Geometry: final body of the model. Coordinates: model frame, mm. Face numbers are marked on the shaded views. A direction names the side the tool comes from. Give positions to 0.01 mm unless a question says otherwise; leave off trailing zeros. Loops run counter-clockwise (first coordinate to the right, second up) from the corner with the lowest first, then second, coordinate; pieces in that order, holes last. Notation, with made-up numbers: (-38, 9) -> (11, 9) arc R31 ccw to (11, 36) -> close; hole circle Ø5 at (42.5, 86). An arc over 180 degrees is marked (long way). One line per item, written item: value. Start each with the question number.
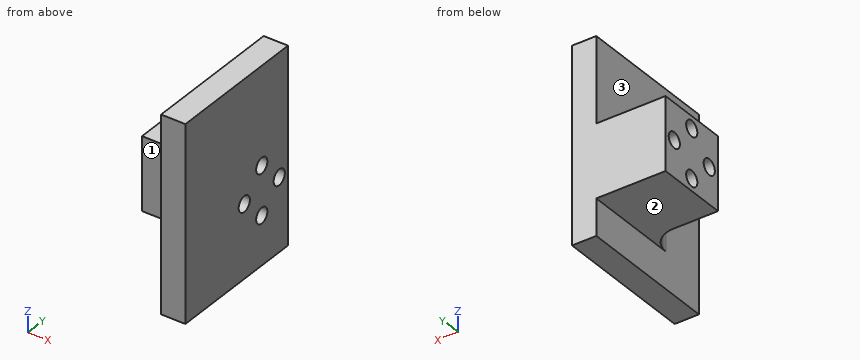
from build123d import *

# Parameters (mm, degrees)
BOSS_EXTRUDE1_DEPTH     = 5
CUT_EXTRUDE1_DEPTH      = 114.468057179
CUT_EXTRUDE1_DEPTH_BACK = 114.468057179
SKETCH3_R               = 1.6
SKETCH4_R               = 2.55
CUT_EXTRUDE2_DEPTH      = 10
SKETCH5_R               = 1.55
CUT_EXTRUDE3_DEPTH      = 114.468057179
SKETCH6_R               = 1.55
CUT_EXTRUDE4_DEPTH      = 114.468057179
SKETCH7_W               = 23
SKETCH7_H               = 110
BOSS_EXTRUDE2_DEPTH     = 5
SKETCH9_W               = 5
SKETCH9_H               = 40
BOSS_EXTRUDE4_DEPTH     = 33
SKETCH11_W              = 12
SKETCH11_H              = 12
CUT_EXTRUDE5_DEPTH      = 50
SKETCH12_R              = 1.6
CUT_EXTRUDE6_DEPTH      = 50
BOSS_EXTRUDE5_START     = 14.25
SKETCH13_W              = 15
SKETCH13_H              = 15
SKETCH13_R              = 1.6
BOSS_EXTRUDE5_DEPTH     = 14.25
SKETCH15_W              = 89.5
SKETCH15_H              = 3.65
CUT_EXTRUDE9_DEPTH      = 153.144667997
SKETCH18_W              = 13
SKETCH18_H              = 110
CUT_EXTRUDE10_DEPTH     = 134.005347637
FILLET5_R               = 5
SKETCH19_R              = 1.55
CUT_EXTRUDE11_DEPTH     = 5
CUT_EXTRUDE12_DEPTH     = 189.758900452


with BuildPart() as part:
    # Sketch1 → Boss-Extrude1 (new body)
    with BuildSketch(Plane(origin=(0, 0, 0), x_dir=(1, 0, 0), z_dir=(0, 1, 0))):
        Polygon((75, 85), (-75, 85), (-75, -25), (-45, -45), (-45, -80), (45, -80), (45, -45), (75, -25), align=None)
        Polygon((-18.5, -10), (-18.5, 10), (-7.5, 10), (-7.5, 50), (7.5, 50), (7.5, 10), (18.5, 10), (18.5, -10), align=None, mode=Mode.SUBTRACT)
    extrude(amount=BOSS_EXTRUDE1_DEPTH)

    # Sketch3 → Cut-Extrude1 (cut, two sides: drawn at the far end of the back side and taken through both)
    with BuildSketch(Plane(origin=(0, 5, 0), x_dir=(1, 0, 0), z_dir=(0, 1, 0)).offset(-CUT_EXTRUDE1_DEPTH_BACK)):
        with Locations(Location((-35, 20, 0), (0, 0, 270))):
            Circle(SKETCH3_R)
        with Locations(Location((-35, -20, 0), (0, 0, 270))):
            Circle(SKETCH3_R)
        with Locations(Location((35, -20, 0), (0, 0, 270))):
            Circle(SKETCH3_R)
        with Locations(Location((35, 20, 0), (0, 0, 270))):
            Circle(SKETCH3_R)
    extrude(amount=CUT_EXTRUDE1_DEPTH + CUT_EXTRUDE1_DEPTH_BACK, mode=Mode.SUBTRACT)

    # Sketch4 → Cut-Extrude2 (cut)
    with BuildSketch(Plane(origin=(0, 5, 0), x_dir=(1, 0, 0), z_dir=(0, 1, 0))):
        with Locations(Location((-65, 66, 0), (0, 0, 270))):
            Circle(SKETCH4_R)
        with Locations(Location((65, -4, 0), (0, 0, 270))):
            Circle(SKETCH4_R)
        with Locations(Location((-65, -4, 0), (0, 0, 270))):
            Circle(SKETCH4_R)
        with Locations(Location((65, 66, 0), (0, 0, 270))):
            Circle(SKETCH4_R)
    extrude(amount=-CUT_EXTRUDE2_DEPTH, mode=Mode.SUBTRACT)

    # Sketch5 → Cut-Extrude3 (cut, through all)
    with BuildSketch(Plane(origin=(0, 5, 0), x_dir=(1, 0, 0), z_dir=(0, 1, 0))):
        with Locations(Location((-39, -75, 0), (0, 0, 270))):
            Circle(SKETCH5_R)
        with Locations(Location((39, -75, 0), (0, 0, 90))):
            Circle(SKETCH5_R)
        with Locations(Location((-39, -50, 0), (0, 0, 270))):
            Circle(SKETCH5_R)
        with Locations(Location((39, -50, 0), (0, 0, 90))):
            Circle(SKETCH5_R)
    extrude(amount=-CUT_EXTRUDE3_DEPTH, mode=Mode.SUBTRACT)

    # Sketch6 → Cut-Extrude4 (cut, through all)
    with BuildSketch(Plane(origin=(0, 5, 0), x_dir=(1, 0, 0), z_dir=(0, 1, 0))):
        with Locations(Location((62.5, 80, 0), (0, 0, 270))):
            Circle(SKETCH6_R)
        with Locations(Location((-62.5, 80, 0), (0, 0, 90))):
            Circle(SKETCH6_R)
    extrude(amount=-CUT_EXTRUDE4_DEPTH, mode=Mode.SUBTRACT)

    # Sketch7 → Boss-Extrude2 (add)
    with BuildSketch(Plane(origin=(0, 5, 0), x_dir=(1, 0, 0), z_dir=(0, 1, 0))):
        with Locations((-86.5, 30)):
            Rectangle(SKETCH7_W, SKETCH7_H)
        with Locations((86.5, 30)):
            Rectangle(SKETCH7_W, SKETCH7_H)
    extrude(amount=-BOSS_EXTRUDE2_DEPTH)

    # Sketch9 → Boss-Extrude4 (add)
    with BuildSketch(Plane(origin=(0, 5, 0), x_dir=(1, 0, 0), z_dir=(0, 1, 0))):
        with Locations((-42.25, -5)):
            Rectangle(SKETCH9_W, SKETCH9_H)
        with Locations((42.25, -5)):
            Rectangle(SKETCH9_W, SKETCH9_H)
    extrude(amount=BOSS_EXTRUDE4_DEPTH)

    # Sketch11 → Cut-Extrude5 (cut)
    with BuildSketch(Plane(origin=(0, 5, 0), x_dir=(1, 0, 0), z_dir=(0, 1, 0))):
        with Locations((-67, 18.305755671)):
            Rectangle(SKETCH11_W, SKETCH11_H)
        with Locations((67, 18.305755671)):
            Rectangle(SKETCH11_W, SKETCH11_H)
    extrude(amount=-CUT_EXTRUDE5_DEPTH, mode=Mode.SUBTRACT)

    # Sketch12 → Cut-Extrude6 (cut)
    with BuildSketch(Plane.ZY.offset(44.75)):
        with Locations((0, 31.85)):
            Circle(SKETCH12_R)
        with Locations((5, 26.85)):
            Circle(SKETCH12_R)
        with Locations((0, 21.85)):
            Circle(SKETCH12_R)
        with Locations((-5, 26.85)):
            Circle(SKETCH12_R)
    cut_extrude6 = extrude(amount=-CUT_EXTRUDE6_DEPTH, mode=Mode.SUBTRACT)

    # Sketch13 → Boss-Extrude5 (add)
    with BuildSketch(Plane.ZY.offset(44.75).offset(BOSS_EXTRUDE5_START)):
        with Locations((0, 26.85)):
            Rectangle(SKETCH13_W, SKETCH13_H)
        with Locations((0, 31.85)):
            Circle(SKETCH13_R, mode=Mode.SUBTRACT)
        with Locations((5, 26.85)):
            Circle(SKETCH13_R, mode=Mode.SUBTRACT)
        with Locations((-5, 26.85)):
            Circle(SKETCH13_R, mode=Mode.SUBTRACT)
        with Locations((0, 21.85)):
            Circle(SKETCH13_R, mode=Mode.SUBTRACT)
    boss_extrude5 = extrude(amount=-BOSS_EXTRUDE5_DEPTH)

    # Mirror2: Cut-Extrude6 across plane
    add(cut_extrude6.mirror(Plane.ZY), mode=Mode.SUBTRACT)

    # Mirror3: Boss-Extrude5 across plane
    add(boss_extrude5.mirror(Plane.ZY))

    # Sketch15 → Cut-Extrude9 (cut, through all)
    with BuildSketch(Plane.XY.offset(25)):
        with Locations((0, 36.175)):
            Rectangle(SKETCH15_W, SKETCH15_H)
    extrude(amount=-CUT_EXTRUDE9_DEPTH, mode=Mode.SUBTRACT)

    # Sketch18 → Cut-Extrude10 (cut, through all)
    with BuildSketch(Plane(origin=(0, 5, 0), x_dir=(1, 0, 0), z_dir=(0, 1, 0))):
        with Locations((-91.5, 30)):
            Rectangle(SKETCH18_W, SKETCH18_H)
        with Locations((91.5, 30)):
            Rectangle(SKETCH18_W, SKETCH18_H)
    extrude(amount=-CUT_EXTRUDE10_DEPTH, mode=Mode.SUBTRACT)

    # Fillet5
    fillet5_edges = [part.edges().sort_by_distance(p)[0] for p in [
        (-44.75, 19.35, 0),
        (44.75, 19.35, 0),
    ]]
    fillet(fillet5_edges, radius=FILLET5_R)

    # Sketch19 → Cut-Extrude11 (cut)
    with BuildSketch(Plane(origin=(0, 5, 0), x_dir=(1, 0, 0), z_dir=(0, 1, 0))):
        with Locations(Location((55, 34.5, 0), (0, 0, 270))):
            Circle(SKETCH19_R)
        with Locations(Location((25, 34.5, 0), (0, 0, 270))):
            Circle(SKETCH19_R)
        with Locations(Location((25, 44.5, 0), (0, 0, 270))):
            Circle(SKETCH19_R)
        with Locations(Location((55, 44.5, 0), (0, 0, 270))):
            Circle(SKETCH19_R)
    cut_extrude11 = extrude(amount=-CUT_EXTRUDE11_DEPTH, mode=Mode.SUBTRACT)

    # Mirror4: Cut-Extrude11 across plane
    add(cut_extrude11.mirror(Plane.ZY), mode=Mode.SUBTRACT)

    # Sketch21 → Cut-Extrude12 (cut, through all)
    with BuildSketch(Plane.XY.offset(80)):
        Polygon((-45, 5), (-45, 0), (45, 0), (45, 5), (39.75, 5), align=None)
        Polygon((39.75, 5), (45, 5), (59, 5), (59, 34.35), (39.75, 34.35), align=None)
        Polygon((45, 5), (45, 0), (85, 0), (85, 5), (59, 5), align=None)
    extrude(amount=-CUT_EXTRUDE12_DEPTH, mode=Mode.SUBTRACT)


with BuildPart() as cut_extrude12_kept_piece:
    # of the separate pieces the step leaves, the one the design keeps (cut_extrude12_pieces_kept)
    add(part.part.solids().sort_by_distance((-44.75, 34.35, 7.5))[0])


solid = cut_extrude12_kept_piece.part
Item 1: Pin query (flat end, axial travel): pin 1 (4.5 mm diameter, centred on x = -53, z = -2.5, fed in from -Y); pin 2 (7 mm diameter, centred on x = -55.5, y = 25.5, fed in from -Z); pin 3 (1.5 mm diameter, centred on x = -55.5, y = 24, fed in from +Z). Return the tip coordinate at first contact, or that it passes through.
Item 2: Section A-A, the plane z = 0. Output: boundary loops of the cut face in (x, y).
Item 3: Access query for the marked faces 1, 2 and 3. Directions: +Z, -Z, +X, -X, +Y, -Y. A direction counts if a zero-diameter tool reaches every point of the face in a straight line with its end or side. Return the directions, or none.
Item 4: Section C-C, the plane x = -43.25. Output: boundary loops of the cut face in (y, z).
Item 5: Ray query, line 1 along Z through (x, y) = (-47.25, 27.75); line 2 along Z through (x, y) = (-43.5, 28.25); line 3 along X through (y, z) = (25, 10). Return the intervals inside material, ascending. Write a range as [from, to].
Item 6: Section B-B, the plane y = 26.85. Output: boundary loops of the cut face in (x, z), then the cut area to 3 significant figures.
Item 7: Section D-D, the plane y = 31.85. Output: boundary loops of the cut face in (x, z), then the cut area to 3 significant figures.
Geometry check:
1. pin 1: stops at y = 19.35
1. pin 2: stops at z = -7.5
1. pin 3: stops at z = 7.5
2. outline: (-59, 19.35) -> (-49.75, 19.35) arc R5 cw to (-44.75, 14.35) -> (-44.75, 5) -> (-39.75, 5) -> (-39.75, 20.25) -> (-59, 20.25) -> close; (-59, 23.45) -> (-39.75, 23.45) -> (-39.75, 30.25) -> (-59, 30.25) -> close; (-59, 33.45) -> (-39.75, 33.45) -> (-39.75, 34.35) -> (-59, 34.35) -> close
3. face 1: +Z, -Z, -X, -Y
3. face 2: -Z, -X, +Y, -Y
3. face 3: -X, -Y
4. outline: (5, -15) -> (34.35, -15) -> (34.35, 25) -> (5, 25) -> close; hole circle Ø3.2 at (21.85, 0); hole circle Ø3.2 at (26.85, -5); hole circle Ø3.2 at (26.85, 5); hole circle Ø3.2 at (31.85, 0)
5. line 1: z = [-7.5, -6.32], [-3.68, 3.68], [6.32, 7.5]
5. line 2: z = [-15, -5.77], [-4.23, 4.23], [5.77, 25]
5. line 3: x = [-44.75, -39.75]
6. outline: (-59, -7.5) -> (-44.75, -7.5) -> (-44.75, -15) -> (-39.75, -15) -> (-39.75, -6.6) -> (-59, -6.6) -> close; (-59, -3.4) -> (-39.75, -3.4) -> (-39.75, 3.4) -> (-59, 3.4) -> close; (-59, 6.6) -> (-39.75, 6.6) -> (-39.75, 25) -> (-44.75, 25) -> (-44.75, 7.5) -> (-59, 7.5) -> close
6. area: 291 mm2
7. outline: (-59, -7.5) -> (-44.75, -7.5) -> (-44.75, -15) -> (-39.75, -15) -> (-39.75, -1.6) -> (-59, -1.6) -> close; (-59, 1.6) -> (-39.75, 1.6) -> (-39.75, 25) -> (-44.75, 25) -> (-44.75, 7.5) -> (-59, 7.5) -> close
7. area: 352 mm2
